Here's how the part is built. I have some questions about the finished solid (model axes, mm). A direction names the side the tool comes from. Coordinates: 2 decimals unless noted, no trailing zeros. Write each loop counter-clockwise with the first axis right and the second up, starting at its lowest first coordinate (ties: lowest second). Pieces come first, ordered by that corner, then holes. Notation, with made-up numbers: M 23.25,17.25 L 44.25,17.25 A17 cw 44.25,30.25 Z; hole C 52,81.5 d3. An arc over 180 degrees is marked long. Use a Markdown table: item, result.
```python
from build123d import *

# Parameters (mm, degrees)
F1_DEPTH      = 30
F3_DEPTH      = 10
F3_DEPTH_BACK = 10
F5_DEPTH      = 30.001
F6_R          = 2.5
F7_DEPTH      = 5
F8_DEPTH      = 10
F10_R         = 2.5
F11_DEPTH     = 16
F12_W         = 40
F12_H         = 10
F13_DEPTH     = 300
F16_DEPTH     = 20


with BuildPart() as f1:
    # F0 (on Top) → F1 (new body)
    with BuildSketch(Plane.XY):
        Polygon((0, -123.1), (0, 0), (0, 123.1), (-1628.22, 123.1), (-1628.22, -123.1), align=None)
    extrude(amount=-F1_DEPTH)

    # F2 (on Front) → F3 (join, two sides)
    with BuildSketch(Plane.XZ) as f3_sk:
        with BuildLine():
            Line((-196.45, 0), (-82.53, 0))
            Line((-82.53, 0), (-82.53, 20))
            ThreePointArc((-82.53, 20), (-196.45, 133.92), (-310.37, 20))
            Line((-310.37, 20), (-310.37, 0))
            Line((-310.37, 0), (-196.45, 0))
        make_face()
    extrude(amount=F3_DEPTH)
    extrude(f3_sk.sketch, amount=-F3_DEPTH_BACK)

    # F4 (on Top) → F5 (cut, through all)
    with BuildSketch(Plane.XY):
        with BuildLine():
            Line((-449.25, 12), (-460.75, 12))
            Line((-460.75, 12), (-472.25, 12))
            Line((-472.25, 12), (-472.25, -12))
            Line((-472.25, -12), (-449.25, -12))
            ThreePointArc((-449.25, -12), (-437.25, 0), (-449.25, 12))
        make_face()
    extrude(amount=-F5_DEPTH, mode=Mode.SUBTRACT)

    # F6 (on Top) → F7 (cut)
    with BuildSketch(Plane.XY):
        Polygon((-167.325, 123.1), (-196.45, 123.1), (-225.575, 123.1), (-225.575, 103.1), (-167.325, 103.1), align=None)
        with Locations((-217.075, 113.1)):
            Circle(F6_R, mode=Mode.SUBTRACT)
        with Locations((-175.825, 113.1)):
            Circle(F6_R, mode=Mode.SUBTRACT)
        Polygon((-167.325, -123.1), (-167.325, -103.1), (-225.575, -103.1), (-225.575, -123.1), (-196.45, -123.1), align=None)
        with Locations((-217.075, -113.1)):
            Circle(F6_R, mode=Mode.SUBTRACT)
        with Locations((-175.825, -113.1)):
            Circle(F6_R, mode=Mode.SUBTRACT)
    extrude(amount=-F7_DEPTH, mode=Mode.SUBTRACT)

    # F8 (cut): faces of the model
    f8_faces = [f1.faces().sort_by_distance(p)[0] for p in [
        (-175.825, 113.1, 0),
        (-217.075, 113.1, 0),
        (-175.825, -113.1, 0),
        (-217.075, -113.1, 0),
    ]]
    extrude(f8_faces, amount=-F8_DEPTH, mode=Mode.SUBTRACT)

    # F10 (on offset) → F11 (cut)
    with BuildSketch(Plane.XY.offset(-30)):
        with Locations((-502.25, -10)):
            Circle(F10_R)
        with Locations((-502.25, 10)):
            Circle(F10_R)
    extrude(amount=F11_DEPTH, mode=Mode.SUBTRACT)

    # F12 (on offset) → F13 (join)
    with BuildSketch(Plane.XY.offset(-30)):
        Polygon((-216.45, -123.1), (-196.45, -123.1), (-176.45, -123.1), (-176.45, -103.1), (-216.45, -103.1), align=None)
        Polygon((-216.45, 103.1), (-176.45, 103.1), (-176.45, 123.1), (-196.45, 123.1), (-216.45, 123.1), align=None)
        with Locations((-1308.21, 5)):
            Rectangle(F12_W, F12_H)
        with Locations((-1308.21, -5)):
            Rectangle(F12_W, F12_H)
    extrude(amount=-F13_DEPTH)

    # F15 (on offset) → F16 (join)
    with BuildSketch(Plane(origin=(0, 0, -330), x_dir=(1, 0, 0), z_dir=(0, 0, -1))):
        Polygon((0, -123.1), (0, 0), (0, 123.1), (-1628.22, 123.1), (-1628.22, -123.1), align=None)
    extrude(amount=-F16_DEPTH)


solid = f1.part
```
1. Will these pins go through, and if not, where does the flat tip stop? pin 1 Ø10 at (x, z) = (-226.5, 80) entering from -Y; pin 2 Ø3 at (y, z) = (8.5, 51.5) entering from +X; pin 3 Ø16 at (y, z) = (-113.5, -119.5) entering from +X.
Answers follow:
| item | result |
|---|---|
| pin 1 | stops at y = -10 |
| pin 2 | stops at x = -86.55 |
| pin 3 | stops at x = -176.45 |
2. Suppose I cut it at D-D on z = -132. Write out the boundary of the cut face in (x, y), and give its area (3 significant figures).
Answers follow:
| item | result |
|---|---|
| outline | M -1328.21,-10 L -1288.21,-10 L -1288.21,10 L -1328.21,10 Z; M -216.45,-123.1 L -176.45,-123.1 L -176.45,-103.1 L -216.45,-103.1 Z; M -216.45,103.1 L -176.45,103.1 L -176.45,123.1 L -216.45,123.1 Z |
| area | 2,400 mm2 |
3. Suppose I cut it at C-C on x = -929. Write out the boundary of the cut face in (y, z).
Answers follow:
| item | result |
|---|---|
| outline | M -123.1,-330 L 123.1,-330 L 123.1,-310 L -123.1,-310 Z; M -123.1,-30 L 123.1,-30 L 123.1,0 L -123.1,0 Z |
4. Which directions (+Z, -Z, +X, -X, +Y, -Y) give clear straight access to the entire face, cutting with the end or side of a thin tool? Please do faces 4 (the face through (-1308, 10, -168)), 5 (the face through (-196, -103.1, -168)), 6 (the face through (-198, -10, 53)).
Answers follow:
| item | result |
|---|---|
| face 4 | +X, -X, +Y |
| face 5 | +X, -X |
| face 6 | +Z, +X, -X, -Y |
5. Suppose I cut it at B-B on y = -66. Write out the boundary of the cut face in (x, z).
Answers follow:
| item | result |
|---|---|
| outline | M -1628.22,-330 L 0,-330 L 0,-310 L -1628.22,-310 Z; M -1628.22,-30 L 0,-30 L 0,0 L -1628.22,0 Z |
6. Suppose I cut it at A-A on x = -196.45. Write out the boundary of the cut face in (y, z).
Answers follow:
| item | result |
|---|---|
| outline | M -123.1,-330 L 123.1,-330 L 123.1,-5 L 103.1,-5 L 103.1,0 L 10,0 L 10,133.92 L -10,133.92 L -10,0 L -103.1,0 L -103.1,-5 L -123.1,-5 Z; hole M -103.1,-310 L 103.1,-310 L 103.1,-30 L -103.1,-30 Z |
7. I need wall thicknesses on probe 1 along Z at (x, y) = (-1343, -75.5); probe 2 along Z at (x, y) = (-455, 6); probe 3 along X at (y, z) = (6.5, 27). Which ranges of each line are inside material? Lowest first, please.
Answers follow:
| item | result |
|---|---|
| probe 1 | z = -330 to -310, -30 to 0 |
| probe 2 | z = -330 to -310 |
| probe 3 | x = -310.15 to -82.75 |
8. We'd pull the mould along Y, two halves only. Please class faces 1 (the face through (-826, -2, -330)), 2 (the face through (-197, 103.1, -168)), 3 (the face through (-198, 10, 53)): +Y half, -Y half, draft (parallel to the pull), parting line (faces both ways), or undercut.
Answers follow:
| item | result |
|---|---|
| face 1 | draft |
| face 2 | undercut |
| face 3 | +Y half |
